The model under review builds one solid part; all positions refer to its coordinate system, in mm. Face numbers are marked on the shaded views. A direction names the side the tool comes from. Give positions to 0.01 mm unless a question says otherwise; leave off trailing zeros. Order: outer loops, then holes, each group sorted by start corner. A loop starts at its lowest first (then second) coordinate and runs counter-clockwise, first axis right, second up. Notation, with made-up numbers: (79.25, 20.25) - (101.25, 20.25) arc R29 cw to (101.25, 59.25) - close; hole circle Ø11 at (53.5, -6.75). An arc over 180 degrees is marked (long way). Put each result on its own line as item: value.
```python
from build123d import *

# Parameters (mm, degrees)
PCB_DEPTH           = 1
SKETCH2_W           = 11
SKETCH2_H           = 11
SENSOR_DEPTH        = 1
SKETCH3_W           = 7.9
SKETCH3_H           = 6.1
SENSOR_GLASS_DEPTH  = 0.3
SKETCH4_R           = 17
SKETCH4_R_2         = 12.7
MOUNT_BASE_DEPTH    = 3
SKETCH5_R           = 12.7
LOCK_RING_DEPTH     = 4
SKETCH6_R           = 15.5
SKETCH6_R_2         = 12.7
CS_TUBE_DEPTH       = 3
SKETCH7_W           = 21
SKETCH7_H           = 5.5
FFC_CONNECTOR_DEPTH = 2.5
SKETCH8_R           = 1.35
HOLES_DEPTH         = 1


with BuildPart() as part:
    # Sketch1 → PCB (new body)
    with BuildSketch(Plane.XY):
        with BuildLine():
            Line((1, 0), (37, 0))
            ThreePointArc((37, 0), (37.707106781, 0.292893219), (38, 1))
            Line((38, 1), (38, 37))
            ThreePointArc((38, 37), (37.707106781, 37.707106781), (37, 38))
            Line((37, 38), (1, 38))
            ThreePointArc((1, 38), (0.292893219, 37.707106781), (0, 37))
            Line((0, 37), (0, 1))
            ThreePointArc((0, 1), (0.292893219, 0.292893219), (1, 0))
        make_face()
    extrude(amount=PCB_DEPTH)

    # Sketch2 → Sensor (add)
    with BuildSketch(Plane.XY.offset(1)):
        with Locations((19, 19)):
            Rectangle(SKETCH2_W, SKETCH2_H)
    extrude(amount=SENSOR_DEPTH)

    # Sketch3 → Sensor_glass (add)
    with BuildSketch(Plane.XY.offset(2)):
        with Locations((19, 19)):
            Rectangle(SKETCH3_W, SKETCH3_H)
    extrude(amount=SENSOR_GLASS_DEPTH)

    # Sketch4 → Mount_base (add)
    with BuildSketch(Plane.XY.offset(1)):
        with Locations((19, 19)):
            Circle(SKETCH4_R)
        with Locations((19, 19)):
            Circle(SKETCH4_R_2, mode=Mode.SUBTRACT)
    extrude(amount=MOUNT_BASE_DEPTH)

    # Sketch5 → Lock_ring (add)
    with BuildSketch(Plane.XY.offset(4)):
        Polygon((37.5, 19), (36.844820274, 20.404417814), (37.272234301, 21.894037603), (36.405421575, 23.178672013), (36.594545551, 24.716814396), (35.537443632, 25.850033439), (35.483620697, 27.398824245), (34.262258942, 28.352724308), (33.966814396, 29.874027167), (32.611266784, 30.625120065), (32.081475452, 32.081475452), (30.625120065, 32.611266784), (29.874027167, 33.966814396), (28.352724308, 34.262258942), (27.398824245, 35.483620697), (25.850033439, 35.537443632), (24.716814396, 36.594545551), (23.178672013, 36.405421575), (21.894037603, 37.272234301), (20.404417814, 36.844820274), (19, 37.5), (17.595582186, 36.844820274), (16.105962397, 37.272234301), (14.821327987, 36.405421575), (13.283185604, 36.594545551), (12.149966561, 35.537443632), (10.601175755, 35.483620697), (9.647275692, 34.262258942), (8.125972833, 33.966814396), (7.374879935, 32.611266784), (5.918524548, 32.081475452), (5.388733216, 30.625120065), (4.033185604, 29.874027167), (3.737741058, 28.352724308), (2.516379303, 27.398824245), (2.462556368, 25.850033439), (1.405454449, 24.716814396), (1.594578425, 23.178672013), (0.727765699, 21.894037603), (1.155179726, 20.404417814), (0.5, 19), (1.155179726, 17.595582186), (0.727765699, 16.105962397), (1.594578425, 14.821327987), (1.405454449, 13.283185604), (2.462556368, 12.149966561), (2.516379303, 10.601175755), (3.737741058, 9.647275692), (4.033185604, 8.125972833), (5.388733216, 7.374879935), (5.918524548, 5.918524548), (7.374879935, 5.388733216), (8.125972833, 4.033185604), (9.647275692, 3.737741058), (10.601175755, 2.516379303), (12.149966561, 2.462556368), (13.283185604, 1.405454449), (14.821327987, 1.594578425), (16.105962397, 0.727765699), (17.595582186, 1.155179726), (19, 0.5), (20.404417814, 1.155179726), (21.894037603, 0.727765699), (23.178672013, 1.594578425), (24.716814396, 1.405454449), (25.850033439, 2.462556368), (27.398824245, 2.516379303), (28.352724308, 3.737741058), (29.874027167, 4.033185604), (30.625120065, 5.388733216), (32.081475452, 5.918524548), (32.611266784, 7.374879935), (33.966814396, 8.125972833), (34.262258942, 9.647275692), (35.483620697, 10.601175755), (35.537443632, 12.149966561), (36.594545551, 13.283185604), (36.405421575, 14.821327987), (37.272234301, 16.105962397), (36.844820274, 17.595582186), align=None)
        with Locations((19, 19)):
            Circle(SKETCH5_R, mode=Mode.SUBTRACT)
    extrude(amount=LOCK_RING_DEPTH)

    # Sketch6 → CS_tube (add)
    with BuildSketch(Plane.XY.offset(8)):
        with Locations((19, 19)):
            Circle(SKETCH6_R)
        with Locations((19, 19)):
            Circle(SKETCH6_R_2, mode=Mode.SUBTRACT)
    extrude(amount=CS_TUBE_DEPTH)

    # Sketch7 → FFC_connector (add)
    with BuildSketch(Plane.XY):
        with Locations((19, 3.5)):
            Rectangle(SKETCH7_W, SKETCH7_H)
    extrude(amount=-FFC_CONNECTOR_DEPTH)

    # Sketch8 → Holes (cut)
    with BuildSketch(Plane.XY.offset(1)):
        with Locations((4, 4)):
            Circle(SKETCH8_R)
        with Locations((4, 34)):
            Circle(SKETCH8_R)
        with Locations((34, 4)):
            Circle(SKETCH8_R)
        with Locations((34, 34)):
            Circle(SKETCH8_R)
    extrude(amount=-HOLES_DEPTH, mode=Mode.SUBTRACT)


solid = part.part
```
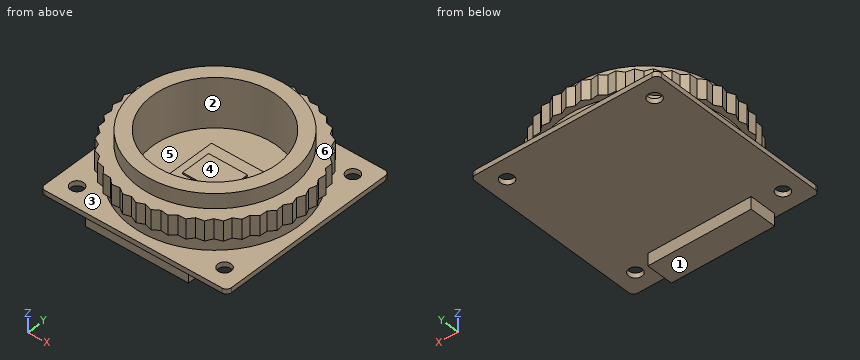
(1) Clearance check with flat-ended pins moving along their axes: pin 1 Ø4 at (x, y) = (7.5, 10) entering from -Z; pin 2 Ø3 at (x, y) = (34, 4) entering from +Z; pin 3 Ø9 at (x, y) = (21, 17) entering from +Z; pin 4 Ø4 at (y, z) = (6, 2) entering from -X. State where each tip first meets the part, or that it passes through.
The answers:
pin 1: z = 0
pin 2: z = 1
pin 3: z = 2.3
pin 4: x = 0
(2) Take a section at B-B, the plane z = -0.5. Write out the cut boundary in (x, y), then the cut area to 4 significant figures.
The answers:
outline: (8.5, 0.75) - (29.5, 0.75) - (29.5, 6.25) - (8.5, 6.25) - close
area: 115.5 mm^2
(3) Take a section at A-A, the plane z = 9. Write out the cut boundary in (x, y).
The answers:
outline: circle Ø31 at (19, 19); hole circle Ø25.4 at (19, 19)
(4) For the marked faces 1, 2 and 3, list the 3-axis set-ups (+Z, -Z, +X, -X, +Y, -Y) from which the entire face can be reached by the end or side of a thin tool; tool diameter is ignored.
The answers:
face 1: -Z, +X, -X, +Y, -Y
face 2: +Z
face 3: none
(5) Wall thickness on L1, parallel to Y at x = 4, z = 0.6; L2, parallel to Z at x = 25, y = 2.5; L3, parallel to Y at x = 19, z = 9.5: over which ranges is each line inside the solid? List them lowest first.
The answers:
L1: 0 to 2.65, 5.35 to 32.65, 35.35 to 38
L2: -2.5 to 1, 4 to 8
L3: 3.5 to 6.3, 31.7 to 34.5
(6) The part is to be moulded in two halves that separate along Y. For the marked faces 4, 5 and 6, say which applies: pulls with the +Y half, pulls with the -Y half, needs draft (parallel to the pull), parting line crosses it, or undercut.
The answers:
face 4: undercut
face 5: undercut
face 6: needs draft
